Design review of the part built by this model. Coordinates are the model's own, in mm. A direction names the side the tool comes from. Give positions to 0.01 mm unless a question says otherwise; leave off trailing zeros. Order: outer loops, then holes, each group sorted by start corner. A loop starts at its lowest first (then second) coordinate and runs counter-clockwise, first axis right, second up. Notation, with made-up numbers: (-32, 44.5) -> (-8, 44.5) arc R5 ccw to (-8, 53.5) -> close; hole circle Ø2 at (78, 7). An arc over 180 degrees is marked (long way). One line per item, written item: value. Start each with the question number.
1) For pin 1 (1 mm diameter, centred on x = -3.5, y = 2, fed in from -Z); pin 2 (6 mm diameter, centred on x = 3, z = 145, fed in from +Y); pin 3 (1.5 mm diameter, centred on y = -6.5, z = 134.5, fed in from +X); pin 4 (4 mm diameter, centred on y = -2.5, z = 85, fed in from +X), all flat-tipped, find the tip position at first contact; note any pin that passes through.
2) Tool access review of faces 1 (the face through (-4.5, -7.4, 255)), 2 (the face through (0, 0, 0)): name each direction out of +Z, -Z, +X, -X, +Y, -Y from which nothing blocks a thin tool from reaching the whole face with its end or side.
3) Consider section A-A (z = 91.5). State the section outline as (x, y) points.
4) Wall thickness on line 1 along Z through (x, y) = (4.75, 0); line 2 along X through (y, z) = (0.5, 209.5); line 3 along Y through (x, z) = (2, 5): over which ranges is each line inside the solid? List them lowest first. Write a range as from..to.
from build123d import *

# Parameters (mm, degrees)
SKETCH1_R               = 6.5
BOSS_EXTRUDE1_DEPTH     = 255
SKETCH2_R               = 10
BOSS_EXTRUDE2_DEPTH     = 5
FILLET1_R               = 2
SKETCH3_R               = 1.5
CUT_EXTRUDE1_DEPTH      = 11.0000001
CUT_EXTRUDE1_DEPTH_BACK = 11


with BuildPart() as part:
    # Sketch1 → Boss-Extrude1 (new body)
    with BuildSketch(Plane.XY):
        Circle(SKETCH1_R)
    extrude(amount=BOSS_EXTRUDE1_DEPTH)

    # Sketch2 → Boss-Extrude2 (add)
    with BuildSketch(Plane.XY.offset(255)):
        Circle(SKETCH2_R)
    extrude(amount=BOSS_EXTRUDE2_DEPTH)

    # Fillet1
    fillet1_edges = [part.edges().sort_by_distance(p)[0] for p in [
        (-6.5, 0, 255),
        (-10, 0, 260),
    ]]
    fillet(fillet1_edges, radius=FILLET1_R)

    # Sketch3 → Cut-Extrude1 (cut, two sides)
    with BuildSketch(Plane(origin=(0, 0, 0), x_dir=(0, 0, -1), z_dir=(1, 0, 0))) as cut_extrude1_sk:
        with Locations((-5, 0)):
            Circle(SKETCH3_R)
    extrude(amount=CUT_EXTRUDE1_DEPTH, mode=Mode.SUBTRACT)
    extrude(cut_extrude1_sk.sketch, amount=-CUT_EXTRUDE1_DEPTH_BACK, mode=Mode.SUBTRACT)


solid = part.part
Checked values:
1. pin 1: stops at z = 0
1. pin 2: stops at y = 6.5
1. pin 3: stops at x = 3.03
1. pin 4: stops at x = 6.48
2. face 1: -Z
2. face 2: -Z, +X, -X, +Y, -Y
3. outline: circle Ø13 at (0, 0)
4. line 1: z = 0..3.5, 6.5..260
4. line 2: x = -6.48..6.48
4. line 3: y = -6.18..-1.5, 1.5..6.18
